```python
from build123d import *

# Parameters (mm, degrees)
SKETCH_1_W          = 180
SKETCH_1_H          = 90
EXTRUDE_1_DEPTH     = 45
SKETCH_3_W          = 84
SKETCH_3_H          = 84
EXTRUDE_3_DEPTH     = 15
EXTRUDE_3_TAPER     = 16
CUT_EXTRUDE_1_DEPTH = 3
FILLET_1_SIZE       = 8


with BuildPart() as part:
    # 草图1 → 凸台-拉伸1 (new, symmetric)
    with BuildSketch(Plane.XY):
        Rectangle(SKETCH_1_W, SKETCH_1_H)
    extrude(amount=EXTRUDE_1_DEPTH, both=True)

    # 草图3 → 凸台-拉伸3 (add)
    with BuildSketch(Plane(origin=(90, 0, 0), x_dir=(0, 0, -1), z_dir=(1, 0, 0))):
        Rectangle(SKETCH_3_W, SKETCH_3_H)
    extrude_3 = extrude(amount=EXTRUDE_3_DEPTH, taper=EXTRUDE_3_TAPER)

    # 镜向2: 凸台-拉伸3 across plane
    add(extrude_3.mirror(Plane(origin=(0, 0, 0), x_dir=(0, 0, 1), z_dir=(1, 0, 0))))

    # 草图5 → 切除-拉伸1 (cut)
    with BuildSketch(Plane(origin=(0, 0, -45), x_dir=(-1, 0, 0), z_dir=(0, 0, -1))):
        Polygon((-90, -25.551009309), (-48.710009236, -25.551009309), (-33.70706091, -10.548060984), (33.70706091, -10.548060984), (48.710009236, -25.551009309), (90, -25.551009309), (90, -30.551009309), (46.638941424, -30.551009309), (31.635993099, -15.548060984), (-31.635993099, -15.548060984), (-46.638941424, -30.551009309), (-90, -30.551009309), align=None)
    cut_extrude_1 = extrude(amount=-CUT_EXTRUDE_1_DEPTH, mode=Mode.SUBTRACT)

    # 镜向3: 切除-拉伸1 across plane
    add(cut_extrude_1.mirror(Plane.XY), mode=Mode.SUBTRACT)

    # 圆角1
    # a fillet whose section is not a circle: 8 mm, written as the material it takes off along each edge
    with BuildSketch(Plane(origin=(110, -45, -45), x_dir=(0, 0, 1), z_dir=(-1, 0, 0)), Plane(origin=(-110, 45, -45), x_dir=(0, 0, 1), z_dir=(1, 0, 0))) as fillet_1_piece_1:
        with BuildLine():
            Bezier((FILLET_1_SIZE, 0), (0, 0), (0, FILLET_1_SIZE), weights=[1, 1, 1])
            Line((0, FILLET_1_SIZE), (0, 0))
            Line((0, 0), (FILLET_1_SIZE, 0))
        make_face()
    extrude(amount=220, mode=Mode.SUBTRACT)
    with BuildSketch(Plane(origin=(-110, 45, 45), x_dir=(0, 0, -1), z_dir=(1, 0, 0)), Plane(origin=(110, -45, 45), x_dir=(0, 0, -1), z_dir=(-1, 0, 0))) as fillet_1_piece_2:
        with BuildLine():
            Bezier((FILLET_1_SIZE, 0), (0, 0), (0, -FILLET_1_SIZE), weights=[1, 1, 1])
            Line((0, -FILLET_1_SIZE), (0, 0))
            Line((0, 0), (FILLET_1_SIZE, 0))
        make_face()
    extrude(amount=220, mode=Mode.SUBTRACT)

    # 草图16 → 旋转1 (revolve)
    with BuildSketch(Plane.XY, mode=Mode.PRIVATE) as revolve_1_sk:
        with BuildLine():
            Line((0, -45), (0, -205.026171576))
            Line((0, -205.026171576), (32.069336895, -205.026171576))
            add(Edge.make_bspline(
                [(15.434694719, -184.505349345), (16.976260644, -200.431842868), (32.069336895, -205.026171576)],
                knots=[0, 0, 0, 1, 1, 1], degree=2))
            Line((15.434694719, -184.505349345), (15.434694719, -45))
            Line((15.434694719, -45), (0, -45))
        make_face()
    revolve(revolve_1_sk.sketch.rotate(Axis((0, -45, 0), (0, -1, 0)), 180), axis=Axis((0, -45, 0), (0, -1, 0)))


solid = part.part
```
Build history of the part. All positions in model axes, mm. A direction names the side the tool comes from. Round coordinates to 2 decimals unless told otherwise and drop trailing zeros. Write each loop counter-clockwise with the first axis right and the second up, starting at its lowest first coordinate (ties: lowest second). Pieces come first, ordered by that corner, then holes.
1) Drill centre lines: probe 1 along X at (y, z) = (-42.5, 41.5); probe 2 along X at (y, z) = (-96.5, -0.5); probe 3 along Y at (x, z) = (-44, 35). Where is each one in solid material? Low to high.
2) Band-saw the part on A-A, the plane y = -56.5. List the corners of the cut face in (x, z).
3) Pin check, flat tips, straight feed: pin 1 (1.5 mm diameter, centred on x = -73.5, z = -43, fed in from -Y); pin 2 (0.9 mm diameter, centred on x = -71.5, z = 44, fed in from -Y); pin 3 (1.5 mm diameter, centred on x = 81, y = -39.5, fed in from -Z). Stop position of each tip, or through.
4) 3-axis set-ups, long thin cutter, end or side, ignore diameter. For faces 1 (the flat face through (-39.24, -23.15, 43.52)), 2 (the flat face through (41.31, -18.15, -43.52)), 3 (the flat face through (-90, 44, 0)), 4 (the flat face through (-1, 6, 45)), 5 (the flat face through (90, 44, 0)): which of +Z, -Z, +X, -X, +Y, -Y reach the whole face in a straight line?
5) Mould opens along Y. For faces 6 (the flat face through (-1, -29, -45)), 7 (the flat face through (0, -15, -42)), 8 (the flat face through (-1, 45, 1)) say: +Y half, -Y half, draft (parallel to the pull), parting line (faces both ways), or undercut.
Ans:
1. probe 1: x = -90 to 90
1. probe 2: x = -15.43 to 15.43
1. probe 3: y = -45 to 45
2. outline: circle Ø30.87 at (0, 0)
3. pin 1: stops at y = -43.63
3. pin 2: stops at y = -42.36
3. pin 3: stops at z = -44.89
4. face 1: +Z
4. face 2: -Z
4. face 3: -X, +Y
4. face 4: +Z, +X, -X, +Y, -Y
4. face 5: +X, +Y
5. face 6: draft
5. face 7: undercut
5. face 8: +Y half
